For this review, take the finished solid that the model builds, in its own axes (mm). A direction names the side the tool comes from. Round coordinates to 2 decimals unless told otherwise and drop trailing zeros. Order: outer loops, then holes, each group sorted by start corner. A loop starts at its lowest first (then second) coordinate and runs counter-clockwise, first axis right, second up. Notation, with made-up numbers: M -14.5,35.25 L 44.5,35.25 A12 ccw 44.5,57.25 Z; hole C -14.75,-26.75 d7. An arc over 180 degrees is marked long. Answer as a JSON object with one key per item and string values.
from build123d import *

# Parameters (mm, degrees)
SKETCH2_W            = 32
SKETCH2_H            = 26
BASE_DEPTH           = 46
SKETCH3_R            = 2
MOUNTING_HOLES_DEPTH = 10
SKETCH4_R            = 3
AXLE_DEPTH           = 10


with BuildPart() as part:
    # Sketch2 → base (new body)
    with BuildSketch(Plane.XY):
        with Locations((16, 13)):
            Rectangle(SKETCH2_W, SKETCH2_H)
    extrude(amount=BASE_DEPTH)

    # Sketch3 → mounting holes (cut)
    with BuildSketch(Plane(origin=(0, 26, 0), x_dir=(1, 0, 0), z_dir=(0, 1, 0))):
        with Locations((5, -5)):
            Circle(SKETCH3_R)
        with Locations((27, -5)):
            Circle(SKETCH3_R)
        with Locations((27, -41)):
            Circle(SKETCH3_R)
        with Locations((5, -41)):
            Circle(SKETCH3_R)
    extrude(amount=-MOUNTING_HOLES_DEPTH, mode=Mode.SUBTRACT)

    # Sketch4 → axle (add)
    with BuildSketch(Plane(origin=(0, 26, 0), x_dir=(1, 0, 0), z_dir=(0, 1, 0))):
        with Locations((16, -15)):
            Circle(SKETCH4_R)
    extrude(amount=AXLE_DEPTH)


solid = part.part
1) Add section B-B on z = 15. State the section outline as (x, y) points, and give its area (3 significant figures).
Geometry check:
{"outline": "M 0,0 L 32,0 L 32,26 L 19,26 L 19,36 L 13,36 L 13,26 L 0,26 Z", "area": "892 mm²"}
2) Add section A-A on x = 16. State the section outline as (y, z) points.
Geometry check:
{"outline": "M 0,0 L 26,0 L 26,12 L 36,12 L 36,18 L 26,18 L 26,46 L 0,46 Z"}
3) Mouldability with a two-part tool opening along Z and no side actions: class faces 1 (the flat face through (16, 13, 0)), 2 (the flat face through (32, 13, 23)), 3 (the cylindrical face through (5, 21, 43)), 4 (the cylindrical face through (28.908, 21.07, 4.399)) as +Z half, -Z half, draft (parallel to the pull), parting line (faces both ways), or undercut.
Geometry check:
{"face 1": "-Z half", "face 2": "draft", "face 3": "undercut", "face 4": "undercut"}
4) Insertion check: P1, Ø3, axis at x = 5, z = 42, coming from the +Y side; P2, Ø2, axis at x = 26.5, z = 5.5, coming from the +Y side. Each pin has a flat end and moves straight along its axis. Give the tip position at first contact, or say it passes through.
Geometry check:
{"P1": "stops at y = 26", "P2": "stops at y = 16"}
5) For L1, parallel to Z at x = 5, y = 21; L2, parallel to X at y = 22, z = 41; L3, parallel to Y at x = 16, z = 37, list the stretches that pass through material, from the lowest coordinate up.
Geometry check:
{"L1": "z = 0 to 3, 7 to 39, 43 to 46", "L2": "x = 0 to 3, 7 to 25, 29 to 32", "L3": "y = 0 to 26"}
6) Machinability: for faces 5 (the flat face through (16, 36, 15)), 6 (the flat face through (27, 16, 5)), which of the approach directions +Z, -Z, +X, -X, +Y, -Y give a long, thin tool a straight path to every point of the face, cutting with its end or side? Answer none if there is none.
Geometry check:
{"face 5": "+Z, -Z, +X, -X, +Y", "face 6": "+Y"}
7) Add section D-D on x = 5. State the section outline as (y, z) points.
Geometry check:
{"outline": "M 0,0 L 26,0 L 26,3 L 16,3 L 16,7 L 26,7 L 26,39 L 16,39 L 16,43 L 26,43 L 26,46 L 0,46 Z"}
8) Add section C-C on z = 5. State the section outline as (x, y) points, and give its area (3 significant figures).
Geometry check:
{"outline": "M 0,0 L 32,0 L 32,26 L 29,26 L 29,16 L 25,16 L 25,26 L 7,26 L 7,16 L 3,16 L 3,26 L 0,26 Z", "area": "752 mm²"}
